Study the drawing (mm; zero at the part's minimum x, y, z) and answer. Round coordinates to 2 decimals unless told otherwise and drop trailing zeros. Loops run counter-clockwise (first coordinate to the right, second up) from the corner with the lowest first, then second, coordinate; pieces in that order, holes last. Notation, with made-up numbers: (52.5, 35) - (105.5, 35) arc R21 cw to (105.5, 43) - close; hole circle Ø8 at (-34.5, 69). An arc over 180 degrees is marked (long way). Use CSV: the item, a comma, the result in double quotes. Start each with the question number.
1. Determine the mould class of the marked faces 1, 2 and 3 for opening direction X: +X half, -X half, draft (parallel to the pull), parting line (faces both ways), or undercut.
2. Find section C-C (x = 27.94). State how many separate pieces and enclosed holes the cut face has.
3. Consider line 1 along X through (y, z) = (1.4, 19.05); line 2 along X through (y, z) = (1.85, 10.16); line 3 along Z through (x, y) = (10.16, 2.65). Determine where each line is inside the solid, lowest interval first.
4. Find section A-A (z = 19.05). Give the vertices of the cut face in (x, y), and give its area (3 significant figures).
5. Find section B-B (y = 3.5). Give the vertices of the cut face in (x, z).
6. Given pin 1 Ø1 at (y, z) = (3, 22.5) entering from -X; pin 2 Ø2 at (y, z) = (1.5, 6) entering from +X (1 decimal), each flat-ended and moving along its own axis, determine where each tip first touches the part or whether it passes through.
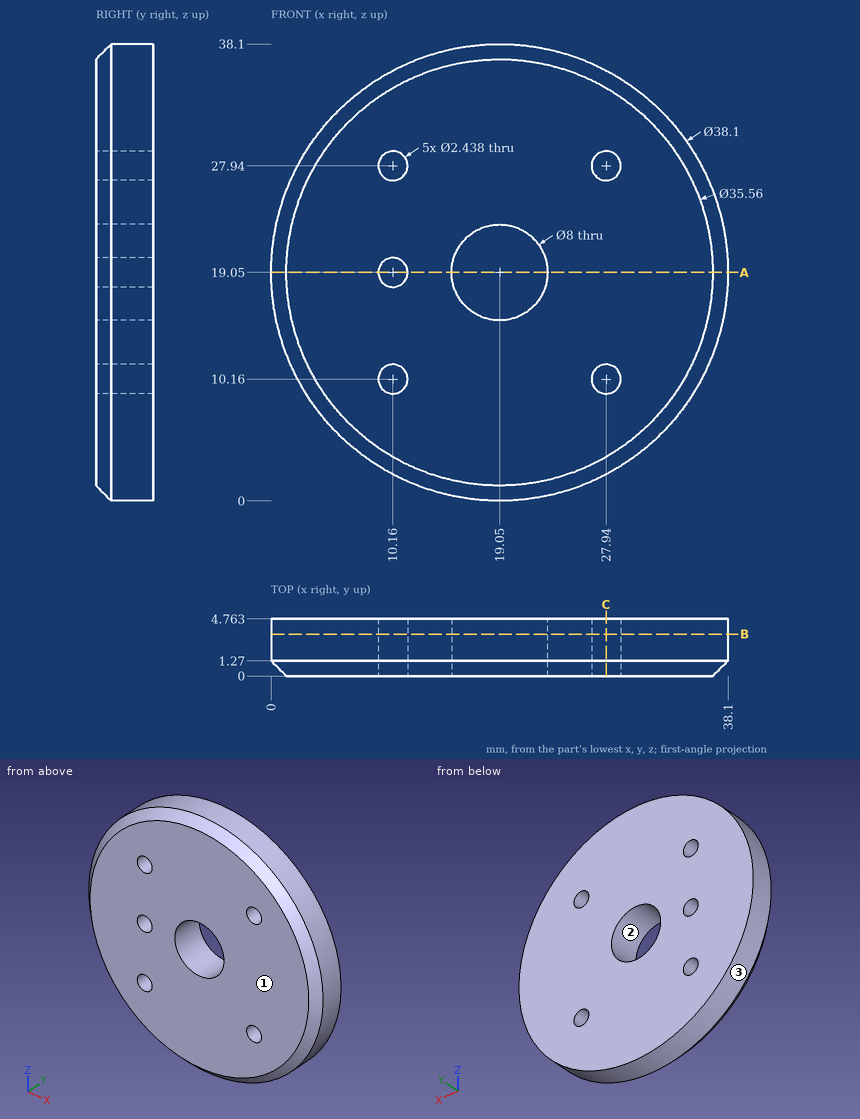
Filled sheet:
1,face 1,"draft"
1,face 2,"undercut"
1,face 3,"parting line"
2,separate pieces,"3"
2,enclosed holes,"0"
3,line 1,"x = 0 to 8.94, 11.38 to 15.05, 23.05 to 38.1"
3,line 2,"x = 2.2 to 8.94, 11.38 to 26.72, 29.16 to 35.9"
3,line 3,"z = 2.2 to 8.94, 11.38 to 17.83, 20.27 to 26.72, 29.16 to 35.9"
4,outline,"(0, 1.27) - (1.27, 0) - (8.94, 0) - (8.94, 4.76) - (0, 4.76) - close; (11.38, 0) - (15.05, 0) - (15.05, 4.76) - (11.38, 4.76) - close; (23.05, 0) - (36.83, 0) - (38.1, 1.27) - (38.1, 4.76) - (23.05, 4.76) - close"
4,area,"130 mm²"
5,outline,"circle Ø38.1 at (19.05, 19.05); hole circle Ø2.44 at (10.16, 10.16); hole circle Ø2.44 at (10.16, 19.05); hole circle Ø2.44 at (10.16, 27.94); hole circle Ø8 at (19.05, 19.05); hole circle Ø2.44 at (27.94, 10.16); hole circle Ø2.44 at (27.94, 27.94)"
6,pin 1,"stops at x = 0.23"
6,pin 2,"stops at x = 33.8"
